Answer from the drawing. Dimensions are ordinates in mm from the lowest x, y and z of the part. Round coordinates to 2 decimals unless told otherwise and drop trailing zeros. Write each loop counter-clockwise with the first axis right and the second up, starting at its lowest first coordinate (ties: lowest second). Pieces come first, ordered by that corner, then holes. Notation, with made-up numbers: M 44.5,-13 L 85.5,-13 A24 cw 85.5,8 Z; hole C 89.5,83.5 d4. An arc over 180 degrees is marked long. One line per item, written item: value. Start each with the question number.
(1) Section A-A (x = 5) is taken. Determine the outline of the cut face in (y, z).
(2) Section C-C (y = 15.75) is taken. Determine the outline of the cut face in (x, z).
(3) Section D-D (x = 2) is taken. Determine the outline of the cut face in (y, z).
(4) Consider probe 1 along Z at (x, y) = (5, 20.25); probe 2 along Z at (x, y) = (6.25, 19.75); probe 3 along X at (y, z) = (16, 4). Determine where each line is inside the solid, lowest interval first.
(5) Given P1, Ø2.5, axis at x = 5, z = 5, coming from the -Y side; P2, Ø3, axis at y = 12.5, z = 2.5, coming from the -X side; P3, Ø1.5, axis at y = 8.5, z = 3, coming from the +X side; P4, Ø3, axis at x = 7, y = 20, coming from the -Z side, each flat-ended and moving along its own axis, determine where each tip first touches the part or whether it passes through.
(6) Section B-B (z = 5) is taken. Determine the outline of the cut face in (x, y).
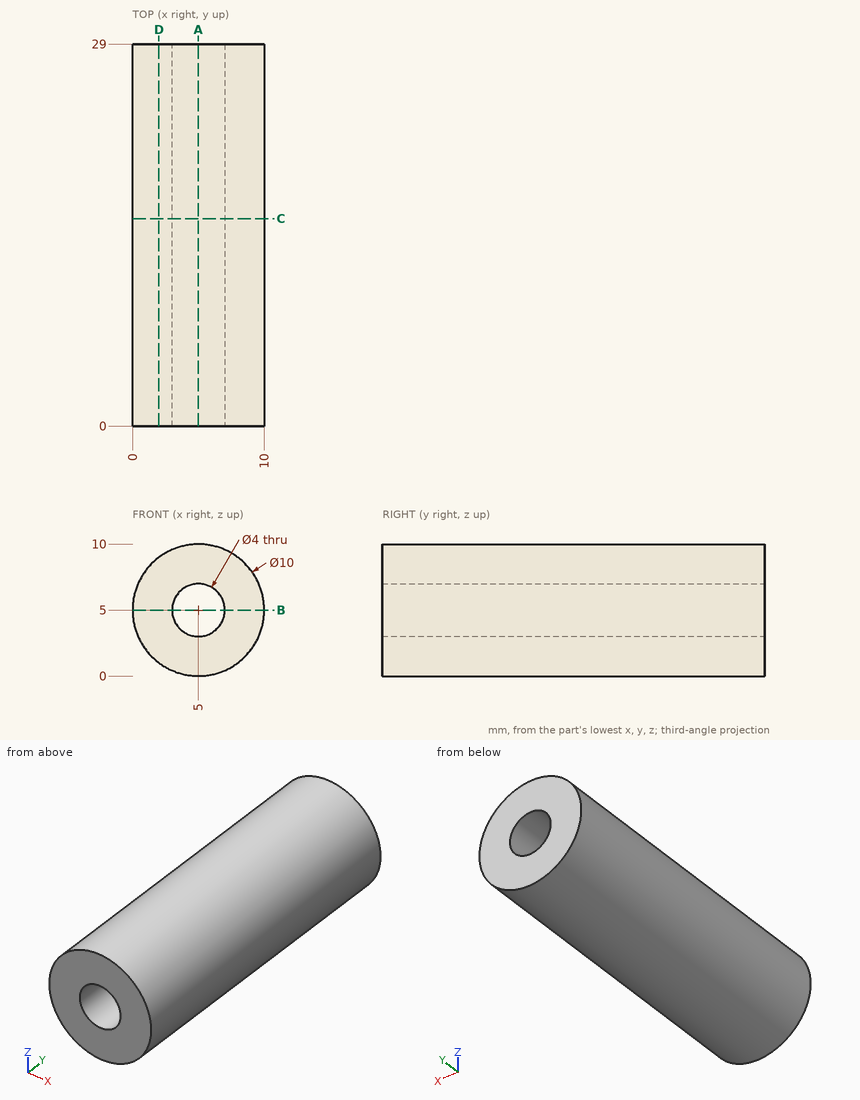
Recorded:
1. outline: M 0,0 L 29,0 L 29,3 L 0,3 Z; M 0,7 L 29,7 L 29,10 L 0,10 Z
2. outline: C 5,5 d10; hole C 5,5 d4
3. outline: M 0,1 L 29,1 L 29,9 L 0,9 Z
4. probe 1: z = 0 to 3, 7 to 10
4. probe 2: z = 0.16 to 3.44, 6.56 to 9.84
4. probe 3: x = 0.1 to 3.27, 6.73 to 9.9
5. P1: passes through
5. P2: stops at x = 0.1
5. P3: stops at x = 9.84
5. P4: stops at z = 0.03
6. outline: M 0,0 L 3,0 L 3,29 L 0,29 Z; M 7,0 L 10,0 L 10,29 L 7,29 Z
